The model under review builds one solid part; all positions refer to its coordinate system, in mm. A direction names the side the tool comes from. Give positions to 0.01 mm unless a question says otherwise; leave off trailing zeros. Loops run counter-clockwise (first coordinate to the right, second up) from the corner with the lowest first, then second, coordinate; pieces in that order, holes last. Notation, with made-up numbers: M -7,41 L 16,41 A12 cw 16,49 Z; hole C 44,1.5 d1. An arc over 180 degrees is marked long. Write item = value, one per line. Start each with the question number.
1. Wall thickness on line 1 along X through (y, z) = (6.75, 45.5); line 2 along Z through (x, y) = (-2, 8.75); line 3 along X through (y, z) = (1.5, 30.5): over which ranges is each line inside the solid? List them lowest first. Write a range as from..to.
2. We need section A-A on x = 45. Give the boundary of the cut face in (y, z), then the cut area to 3 significant figures.
3. For faces 1 (the face through (33.32, 2.46, 27.05)), 2 (the face through (-23, 11, 0)), 3 (the face through (-29.192, 8.796, -31.475)), list the 3-axis set-ups (+Z, -Z, +X, -X, +Y, -Y) from which the entire face can be reached by the end or side of a thin tool; tool diameter is ignored.
4. For pin 1 (3 mm diameter, centred on y = 10, z = -0.5, fed in from +X); pin 2 (4.5 mm diameter, centred on x = 2.5, y = 10, fed in from +Z); pin 3 (5 mm diameter, centred on x = -39, y = 4, fed in from -Z); pin 4 (6 mm diameter, centred on x = 18, z = 0, fed in from -Y), all flat-tipped, find the tip position at first contact; note any pin that passes through.
5. We need section B-B on y = 1.75. Count the separate pieces of the cut face and the enclosed holes in it, then the cut area to 3 significant figures.
6. We need section D-D on x = -7. Give the boundary of the cut face in (y, z).
7. We need section C-C on z = 45. Give the boundary of the cut face in (x, y), then the cut area to 3 significant figures.
from build123d import *

# Parameters (mm, degrees)
SKETCH1_R           = 72.5
BOSS_EXTRUDE1_DEPTH = 12.7
SKETCH2_R           = 2.65
CUT_EXTRUDE1_DEPTH  = 104.314035833
SKETCH3_R           = 5
CUT_EXTRUDE2_DEPTH  = 5
SKETCH4_R           = 2.75
CUT_EXTRUDE3_DEPTH  = 104.314035833
SKETCH7_W           = 46
SKETCH7_H           = 46
CUT_EXTRUDE6_DEPTH  = 4
SKETCH8_R           = 2.25
CUT_EXTRUDE7_DEPTH  = 103.898930995
SKETCH9_R           = 2.75
CUT_EXTRUDE8_DEPTH  = 104.314035833
SKETCH10_R          = 5
CUT_EXTRUDE9_DEPTH  = 4.7


with BuildPart() as part:
    # Sketch1 → Boss-Extrude1 (new body)
    with BuildSketch(Plane(origin=(0, 0, 0), x_dir=(1, 0, 0), z_dir=(0, 1, 0))):
        with Locations(Location((0, 0, 0), (0, 0, 270))):
            Circle(SKETCH1_R)
    extrude(amount=BOSS_EXTRUDE1_DEPTH)

    # Sketch2 → Cut-Extrude1 (cut, through all)
    with BuildSketch(Plane.XZ):
        with Locations(Location((31.819805153, 31.819805153, 0), (0, 0, 270))):
            Circle(SKETCH2_R)
        with Locations(Location((31.819805153, -31.819805153, 0), (0, 0, 270))):
            Circle(SKETCH2_R)
        with Locations(Location((-31.819805153, -31.819805153, 0), (0, 0, 270))):
            Circle(SKETCH2_R)
        with Locations(Location((-31.819805153, 31.819805153, 0), (0, 0, 270))):
            Circle(SKETCH2_R)
    extrude(amount=-CUT_EXTRUDE1_DEPTH, mode=Mode.SUBTRACT)

    # Sketch3 → Cut-Extrude2 (cut)
    with BuildSketch(Plane.XZ):
        with Locations(Location((-31.819805153, 31.819805153, 0), (0, 0, 270))):
            Circle(SKETCH3_R)
        with Locations(Location((31.819805153, 31.819805153, 0), (0, 0, 270))):
            Circle(SKETCH3_R)
        with Locations(Location((31.819805153, -31.819805153, 0), (0, 0, 270))):
            Circle(SKETCH3_R)
        with Locations(Location((-31.819805153, -31.819805153, 0), (0, 0, 270))):
            Circle(SKETCH3_R)
    extrude(amount=-CUT_EXTRUDE2_DEPTH, mode=Mode.SUBTRACT)

    # Sketch4 → Cut-Extrude3 (cut, through all)
    with BuildSketch(Plane.XZ):
        with Locations(Location((13, 45, 0), (0, 0, 270))):
            Circle(SKETCH4_R)
        with Locations(Location((-13, 45, 0), (0, 0, 90))):
            Circle(SKETCH4_R)
        with Locations(Location((45, -13, 0), (0, 0, 270))):
            Circle(SKETCH4_R)
        with Locations(Location((45, 13, 0), (0, 0, 90))):
            Circle(SKETCH4_R)
        with Locations(Location((-13, -45, 0), (0, 0, 270))):
            Circle(SKETCH4_R)
        with Locations(Location((13, -45, 0), (0, 0, 90))):
            Circle(SKETCH4_R)
        with Locations(Location((-45, 13, 0), (0, 0, 270))):
            Circle(SKETCH4_R)
        with Locations(Location((-45, -13, 0), (0, 0, 90))):
            Circle(SKETCH4_R)
    extrude(amount=-CUT_EXTRUDE3_DEPTH, mode=Mode.SUBTRACT)

    # Sketch7 → Cut-Extrude6 (cut)
    with BuildSketch(Plane(origin=(0, 12.7, 0), x_dir=(1, 0, 0), z_dir=(0, 1, 0))):
        Rectangle(SKETCH7_W, SKETCH7_H)
    extrude(amount=-CUT_EXTRUDE6_DEPTH, mode=Mode.SUBTRACT)

    # Sketch8 → Cut-Extrude7 (cut, through all)
    with BuildSketch(Plane(origin=(0, 8.7, 0), x_dir=(1, 0, 0), z_dir=(0, 1, 0))):
        with Locations(Location((15.556349186, 15.556349186, 0), (0, 0, 270))):
            Circle(SKETCH8_R)
        with Locations(Location((-15.556349186, 15.556349186, 0), (0, 0, 90))):
            Circle(SKETCH8_R)
        with Locations(Location((15.556349186, -15.556349186, 0), (0, 0, 90))):
            Circle(SKETCH8_R)
        with Locations(Location((-15.556349186, -15.556349186, 0), (0, 0, 270))):
            Circle(SKETCH8_R)
    extrude(amount=-CUT_EXTRUDE7_DEPTH, mode=Mode.SUBTRACT)

    # Sketch9 → Cut-Extrude8 (cut, through all)
    with BuildSketch(Plane.XZ):
        with Locations(Location((18, 0, 0), (0, 0, 270))):
            Circle(SKETCH9_R)
        with Locations(Location((-18, 0, 0), (0, 0, 90))):
            Circle(SKETCH9_R)
    extrude(amount=-CUT_EXTRUDE8_DEPTH, mode=Mode.SUBTRACT)

    # Sketch10 → Cut-Extrude9 (cut)
    with BuildSketch(Plane(origin=(0, 8.7, 0), x_dir=(1, 0, 0), z_dir=(0, 1, 0))):
        with Locations(Location((-18, 0, 0), (0, 0, 270))):
            Circle(SKETCH10_R)
        with Locations(Location((18, 0, 0), (0, 0, 270))):
            Circle(SKETCH10_R)
    extrude(amount=-CUT_EXTRUDE9_DEPTH, mode=Mode.SUBTRACT)


solid = part.part
Final values:
q1.line_1 = -56.44..-15.7, -10.3..10.3, 15.7..56.44
q1.line_2 = -72.47..-23, 23..72.47
q1.line_3 = -65.77..-36.64, -27..27, 36.64..65.77
q2.outline = M 0,-56.84 L 12.7,-56.84 L 12.7,-15.75 L 0,-15.75 Z; M 0,-10.25 L 12.7,-10.25 L 12.7,10.25 L 0,10.25 Z; M 0,15.75 L 12.7,15.75 L 12.7,56.84 L 0,56.84 Z
q2.area = 1,300 mm²
q3.face_1 = -Y
q3.face_2 = +Y
q3.face_3 = +Y, -Y
q4.pin_1 = 72.5
q4.pin_2 = 72.5
q4.pin_3 = -62.64
q4.pin_4 = 0
q5.separate_pieces = 1
q5.enclosed_holes = 18
q5.area = 15,900 mm²
q6.outline = M 0,-72.16 L 12.7,-72.16 L 12.7,-23 L 8.7,-23 L 8.7,23 L 12.7,23 L 12.7,72.16 L 0,72.16 Z
q7.outline = M -56.84,0 L -15.75,0 L -15.75,12.7 L -56.84,12.7 Z; M -10.25,0 L 10.25,0 L 10.25,12.7 L -10.25,12.7 Z; M 15.75,0 L 56.84,0 L 56.84,12.7 L 15.75,12.7 Z
q7.area = 1,300 mm²
